Build history of the part. All positions in model axes, mm. Face numbers are marked on the shaded views. A direction names the side the tool comes from. Round coordinates to 2 decimals unless told otherwise and drop trailing zeros. Loops run counter-clockwise (first coordinate to the right, second up) from the corner with the lowest first, then second, coordinate; pieces in that order, holes last.
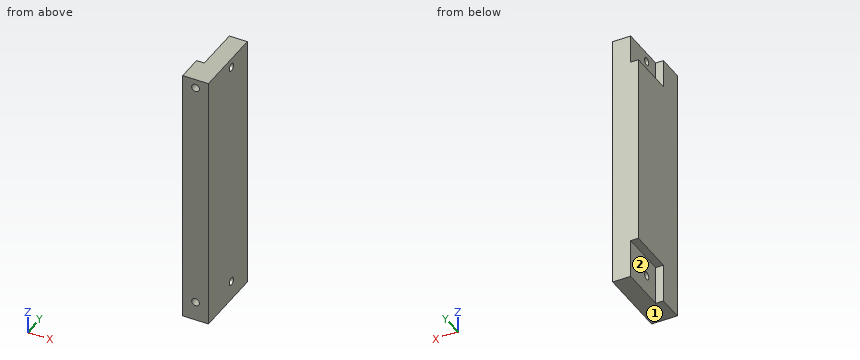
from build123d import *

# Parameters (mm, degrees)
SKETCH_1_W          = 10
SKETCH_1_H          = 28
EXTRUDE_1_DEPTH     = 105
SKETCH_2_R          = 1.5
CUT_EXTRUDE_1_DEPTH = 10
SKETCH_3_R          = 1.5
CUT_EXTRUDE_2_DEPTH = 107.40018797
SKETCH_4_W          = 15
SKETCH_4_H          = 18
CUT_EXTRUDE_3_DEPTH = 3
SKETCH_5_W          = 19.297402577
SKETCH_5_H          = 33.931864009
CUT_EXTRUDE_6_DEPTH = 4


with BuildPart() as part:
    # 草图1 → 凸台-拉伸1 (new body)
    with BuildSketch(Plane.XY):
        Rectangle(SKETCH_1_W, SKETCH_1_H)
    extrude(amount=EXTRUDE_1_DEPTH)

    # 草图2 → 切除-拉伸1 (cut)
    with BuildSketch(Plane.XZ.offset(14)):
        with Locations(Location((0, 97.5, 0), (0, 0, 270))):
            Circle(SKETCH_2_R)
        with Locations(Location((0, 7.5, 0), (0, 0, 270))):
            Circle(SKETCH_2_R)
    extrude(amount=-CUT_EXTRUDE_1_DEPTH, mode=Mode.SUBTRACT)

    # 草图3 → 切除-拉伸2 (cut, through all)
    with BuildSketch(Plane.ZY.offset(5)):
        with Locations(Location((7.5, 2.5, 0), (0, 0, 270))):
            Circle(SKETCH_3_R)
        with Locations(Location((97.5, 2.5, 0), (0, 0, 270))):
            Circle(SKETCH_3_R)
    extrude(amount=-CUT_EXTRUDE_2_DEPTH, mode=Mode.SUBTRACT)

    # 草图4 → 切除-拉伸3 (cut)
    with BuildSketch(Plane.ZY.offset(5)):
        with Locations((7.5, 5)):
            Rectangle(SKETCH_4_W, SKETCH_4_H)
        with Locations((97.5, 5)):
            Rectangle(SKETCH_4_W, SKETCH_4_H)
    extrude(amount=-CUT_EXTRUDE_3_DEPTH, mode=Mode.SUBTRACT)

    # 草图5 → 切除-拉伸6 (cut)
    with BuildSketch(Plane.XY.offset(105)):
        with Locations((1.058128951, -0.39887643)):
            Rectangle(SKETCH_5_W, SKETCH_5_H)
    extrude(amount=-CUT_EXTRUDE_6_DEPTH, mode=Mode.SUBTRACT)


solid = part.part
(1) Slice it at A-A on z = 7.5. List the corners of the cut face in (x, y).
Responses:
outline: (-5, -14) - (-1.5, -14) - (-1.5, -4) - (1.5, -4) - (1.5, -14) - (5, -14) - (5, 1) - (-2, 1) - (-2, -4) - (-5, -4) - close; (-2, 4) - (5, 4) - (5, 14) - (-2, 14) - close
(2) Slice it at C-C on x = -3. List the corners of the cut face in (y, z).
Responses:
outline: (-14, 0) - (-4, 0) - (-4, 15) - (14, 15) - (14, 90) - (-4, 90) - (-4, 101) - (-14, 101) - close
(3) Which spindle directions (+Z, -Z, +X, -X, +Y, -Y) get a long thin tool onto all of the face, cutting with end or side? Do the marked faces 1 and 2. Say none if no direction does.
Responses:
face 1: -Z, +X, -X, +Y, -Y
face 2: -Z, -X, +Y
(4) Slice it at D-D on y = 7. List the corners of the cut face in (x, z).
Responses:
outline: (-5, 15) - (-2, 15) - (-2, 0) - (5, 0) - (5, 101) - (-2, 101) - (-2, 90) - (-5, 90) - close
(5) Probe line 1 (Z direction, x = 1.75, y = 2.5); line 2 (X direction, y = -9.25, z = 97.5); line 3 (Z direction, x = -4.25, y = 1). List the from-to ranges inside material, lowest first.
Responses:
line 1: z = 0 to 6, 9 to 96, 99 to 101
line 2: x = -5 to -1.5, 1.5 to 5
line 3: z = 15 to 90
(6) Pin check, flat tips, straight feed: P1, Ø3.5, axis at y = 2.5, z = 7.5, coming from the -X side; P2, Ø1.8, axis at x = 0, z = 97.5, coming from the -Y side; P3, Ø2.5, axis at x = -4, y = 5, coming from the -Z side. Stop position of each tip, or through.
Responses:
P1: stops at x = -2
P2: stops at y = -4
P3: stops at z = 15
(7) Slice it at B-B on y = 2.5. List the corners of the cut face in (x, z), plus the area to 3 significant figures.
Responses:
outline: (-5, 15) - (-2, 15) - (-2, 9) - (5, 9) - (5, 96) - (-2, 96) - (-2, 90) - (-5, 90) - close; (-2, 0) - (5, 0) - (5, 6) - (-2, 6) - close; (-2, 99) - (5, 99) - (5, 101) - (-2, 101) - close
area: 890 mm2
